Here's the drawing with two shaded views (mm, measured from the low corner). I have some questions. A direction names the side the tool comes from. Give positions to 0.01 mm unless a question says otherwise; leave off trailing zeros. Loops run counter-clockwise (first coordinate to the right, second up) from the corner with the lowest first, then second, coordinate; pieces in that order, holes last.
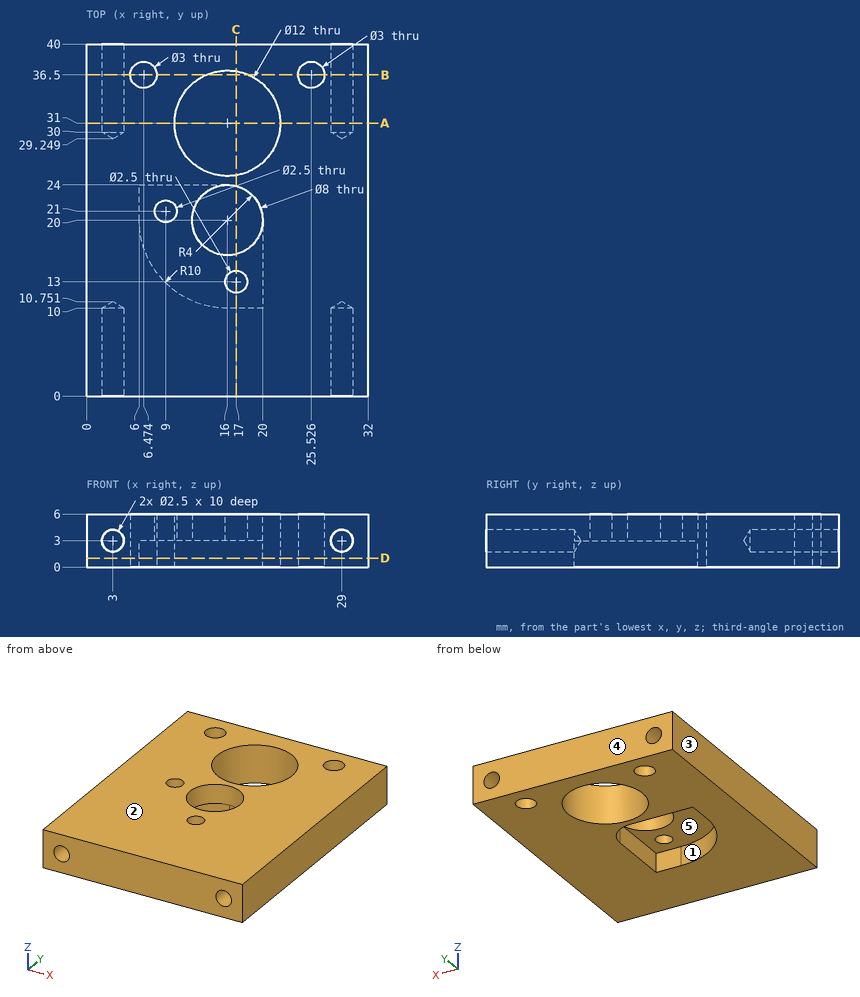
(1) Suppose I cut it at B-B on y = 36.5. List the corners of the cut face in (x, z) for me, plus the area to 3 significant figures.
Returned:
outline: (0, 0) - (4.97, 0) - (4.97, 6) - (0, 6) - close; (7.97, 0) - (13.6, 0) - (13.6, 6) - (7.97, 6) - close; (18.4, 0) - (24.03, 0) - (24.03, 6) - (18.4, 6) - close; (27.03, 0) - (32, 0) - (32, 6) - (27.03, 6) - close; hole circle Ø2.5 at (3, 3); hole circle Ø2.5 at (29, 3)
area: 117 mm2
(2) Thinking about a two-plate mould opening in X: for the marked faces 3, 4 and 5, which applies, pulls with the +X half, pulls with the -X half, needs draft (parallel to the pull), parting line crosses it, or undercut?
Returned:
face 3: pulls with the -X half
face 4: needs draft
face 5: undercut
(3) Please list where these lines run through material, in increasing order: probe 1 along X at (y, z) = (3, 3.3); probe 2 along X at (y, z) = (3.5, 3.9); probe 3 along Y at (x, z) = (12, 2.6) (1 decimal).
Returned:
probe 1: x = 0 to 1.79, 4.21 to 27.79, 30.21 to 32
probe 2: x = 0 to 2.13, 3.87 to 28.13, 29.87 to 32
probe 3: y = 0 to 10.8, 24 to 26.5, 35.5 to 40
(4) Suppose I cut it at A-A on y = 31. List the corners of the cut face in (x, z) for me, plus the area to 3 significant figures.
Returned:
outline: (0, 0) - (10, 0) - (10, 6) - (0, 6) - close; (22, 0) - (32, 0) - (32, 6) - (22, 6) - close; hole circle Ø2.5 at (3, 3); hole circle Ø2.5 at (29, 3)
area: 110 mm2
(5) Suppose I cut it at D-D on z = 1. List the corners of the cut face in (x, y) for me.
Returned:
outline: (0, 0) - (32, 0) - (32, 40) - (0, 40) - close; hole circle Ø3 at (6.47, 36.5); hole (6, 20) arc R10 ccw to (16, 10) - (20, 10) - (20, 20) arc R4 ccw to (16, 24) - (6, 24) - close; hole circle Ø12 at (16, 31); hole circle Ø3 at (25.53, 36.5)
(6) Will these pins go through, and if not, where does the flat tip stop? P1, Ø7, axis at x = 16, y = 20, coming from the -Z side; P2, Ø2, axis at x = 29, z = 3, coming from the -Y side; P3, Ø4, axis at x = 10, y = 18.5, coming from the -Z side.
Returned:
P1: passes through
P2: stops at y = 10.15
P3: stops at z = 3
(7) Which directions (+Z, -Z, +X, -X, +Y, -Y) give clear straight access to the entire face, cutting with the end or side of a thin tool? Please do the marked faces 1 and 2.
Returned:
face 1: -Z
face 2: +Z, +X, -X, +Y, -Y
(8) Suppose I cut it at C-C on x = 17. List the corners of the cut face in (y, z) for me.
Returned:
outline: (0, 0) - (10, 0) - (10, 3) - (11.75, 3) - (11.75, 6) - (0, 6) - close; (14.25, 3) - (16.13, 3) - (16.13, 6) - (14.25, 6) - close; (23.87, 0) - (25.08, 0) - (25.08, 6) - (23.87, 6) - close; (36.92, 0) - (40, 0) - (40, 6) - (36.92, 6) - close
